from build123d import *

# Parameters (mm, degrees)
SKETCH_W        = 38
SKETCH_H        = 20
SKETCH_R        = 2.1
PAD_DEPTH       = 22
SKETCH001_R     = 11.2
POCKET_DEPTH    = 8
SKETCH002_R     = 5.1
SKETCH002_R_2   = 1.75
POCKET001_DEPTH = 20
POCKET002_DEPTH = 3.4


with BuildPart() as part:
    # Sketch → Pad (new body)
    with BuildSketch(Plane.XY):
        with Locations((19, 10)):
            Rectangle(SKETCH_W, SKETCH_H)
        with Locations((4, 15)):
            Circle(SKETCH_R, mode=Mode.SUBTRACT)
        with Locations((4, 5)):
            Circle(SKETCH_R, mode=Mode.SUBTRACT)
        with Locations((34, 15)):
            Circle(SKETCH_R, mode=Mode.SUBTRACT)
        with Locations((34, 5)):
            Circle(SKETCH_R, mode=Mode.SUBTRACT)
    extrude(amount=PAD_DEPTH)

    # Sketch001 (on Face3 of Pad) → Pocket (cut)
    with BuildSketch(Plane.XZ):
        with Locations((19, 11)):
            Circle(SKETCH001_R)
    extrude(amount=-POCKET_DEPTH, mode=Mode.SUBTRACT)

    # Sketch002 (on Face1 of Pocket) → Pocket001 (cut)
    with BuildSketch(Plane(origin=(0, 20, 0), x_dir=(-1, 0, 0), z_dir=(0, 1, 0))):
        with Locations((-19, 11)):
            Circle(SKETCH002_R)
        with Locations((-13.378501, 16.621499)):
            Circle(SKETCH002_R_2)
        with Locations((-24.621499, 5.378501)):
            Circle(SKETCH002_R_2)
        with Locations((-24.621499, 16.621499)):
            Circle(SKETCH002_R_2)
        with Locations((-13.378501, 5.378501)):
            Circle(SKETCH002_R_2)
    extrude(amount=-POCKET001_DEPTH, mode=Mode.SUBTRACT)

    # Sketch003 (on Face4 of Pocket001) → Pocket002 (cut)
    with BuildSketch(Plane.XY.offset(22)):
        Polygon((4, 10.900813), (7.55, 12.950407), (7.55, 17.049593), (4, 19.099187), (0.45, 17.049593), (0.45, 12.950407), align=None)
        Polygon((34, 10.900813), (37.55, 12.950407), (37.55, 17.049593), (34, 19.099187), (30.45, 17.049593), (30.45, 12.950407), align=None)
        Polygon((34, 9.099187), (30.45, 7.049593), (30.45, 2.950407), (34, 0.900813), (37.55, 2.950407), (37.55, 7.049593), align=None)
        Polygon((4, 9.099187), (0.45, 7.049593), (0.45, 2.950407), (4, 0.900813), (7.55, 2.950407), (7.55, 7.049593), align=None)
    extrude(amount=-POCKET002_DEPTH, mode=Mode.SUBTRACT)


solid = part.part
The listing builds one solid part. Answer for the finished solid, in the listing's coordinates (mm). A direction names the side the tool comes from. Round coordinates to 2 decimals unless told otherwise and drop trailing zeros. Order: outer loops, then holes, each group sorted by start corner. A loop starts at its lowest first (then second) coordinate and runs counter-clockwise, first axis right, second up. Notation, with made-up numbers: (6, -18.5) -> (11, -18.5) arc R18 cw to (11, 13.5) -> close; hole circle Ø4 at (55, 50). An arc over 180 degrees is marked (long way). One line per item, written item: value.
Item 1: Find section D-D, the plane z = 17.5. Give the vertices of the cut face in (x, y).
Taken from the geometry:
outline: (0, 0) -> (9.88, 0) -> (9.88, 8) -> (11.86, 8) -> (11.86, 20) -> (0, 20) -> close; (14.89, 8) -> (23.11, 8) -> (23.11, 20) -> (14.89, 20) -> close; (26.14, 8) -> (28.12, 8) -> (28.12, 0) -> (38, 0) -> (38, 20) -> (26.14, 20) -> close; hole circle Ø4.2 at (4, 5); hole circle Ø4.2 at (4, 15); hole circle Ø4.2 at (34, 5); hole circle Ø4.2 at (34, 15)
Item 2: For a pull along X with two mould halves and no side action, classify faces 1 (the flat face through (0, 10, 11)), 2 (the flat face through (2.2, 11.94, 20.32)), 3 (the flat face through (38, 10, 11)) as released by +X, released by -X, zero draft, split by the parting line, or undercut.
Taken from the geometry:
face 1: released by -X
face 2: undercut
face 3: released by +X
Item 3: For faces 4 (the flat face through (19, 10, 22)), 5 (the flat face through (32.2, 11.94, 20.32)), determine the directions among +Z, -Z, +X, -X, +Y, -Y from which every point of the face is accessible in a straight line to the end or side of a thin tool.
Taken from the geometry:
face 4: +Z, +X, -X, +Y, -Y
face 5: +Z
Item 4: Straight lines are drawn through the part: L1, parallel to Y at x = 4, z = 9.5; L2, parallel to X at y = 16.75, z = 20; L3, parallel to X at y = 17.5, z = 20.25. For each, find the intervals that lie inside material, in ascending order.
Taken from the geometry:
L1: y = 0 to 2.9, 7.1 to 12.9, 17.1 to 20
L2: x = 0 to 0.45, 7.55 to 30.45, 37.55 to 38
L3: x = 0 to 1.23, 6.77 to 31.23, 36.77 to 38
Item 5: Find section C-C, the plane y = 5. Give the vertices of the cut face in (x, z).
Taken from the geometry:
outline: (0, 0) -> (1.9, 0) -> (1.9, 18.6) -> (0.45, 18.6) -> (0.45, 22) -> (0, 22) -> close; (6.1, 0) -> (16.89, 0) arc R11.2 cw to (16.89, 22) -> (7.55, 22) -> (7.55, 18.6) -> (6.1, 18.6) -> close; (21.11, 0) -> (31.9, 0) -> (31.9, 18.6) -> (30.45, 18.6) -> (30.45, 22) -> (21.11, 22) arc R11.2 cw to start; (36.1, 0) -> (38, 0) -> (38, 22) -> (37.55, 22) -> (37.55, 18.6) -> (36.1, 18.6) -> close
Item 6: Find section A-A, the plane z = 11. Give the vertices of the cut face in (x, y).
Taken from the geometry:
outline: (0, 0) -> (7.8, 0) -> (7.8, 8) -> (13.9, 8) -> (13.9, 20) -> (0, 20) -> close; (24.1, 8) -> (30.2, 8) -> (30.2, 0) -> (38, 0) -> (38, 20) -> (24.1, 20) -> close; hole circle Ø4.2 at (4, 5); hole circle Ø4.2 at (4, 15); hole circle Ø4.2 at (34, 5); hole circle Ø4.2 at (34, 15)
Item 7: Find section B-B, the plane x = 19. Give the vertices of the cut face in (y, z), then the cut area to 3 significant figures.
Taken from the geometry:
outline: (8, 0) -> (20, 0) -> (20, 5.9) -> (8, 5.9) -> close; (8, 16.1) -> (20, 16.1) -> (20, 22) -> (8, 22) -> close
area: 142 mm2
Item 8: Given P1, Ø5.5, axis at x = 4, y = 15, coming from the +Z side; P2, Ø11, axis at x = 14, z = 10.5, coming from the -Y side; P3, Ø3.5, axis at x = 34, y = 15, coming from the +Z side, each flat-ended and moving along its own axis, determine where each tip first touches the part or whether it passes through.
Taken from the geometry:
P1: stops at z = 18.6
P2: stops at y = 8
P3: passes through
